```python
from build123d import *

# Parameters (mm, degrees)
F1_DEPTH = 2.5
F2_R     = 0.5
F3_DEPTH = 25


with BuildPart() as f1:
    # F0 (on Front) → F1 (new body, symmetric)
    with BuildSketch(Plane.XZ):
        with BuildLine():
            Line((121.261015, -15), (150, -15))
            ThreePointArc((150, -15), (0, 14.918645), (-150, -15))
            Line((-150, -15), (-121.261015, -15))
            ThreePointArc((-121.261015, -15), (0, 4.565027), (121.261015, -15))
        make_face()
    extrude(amount=F1_DEPTH, both=True)

    # F2 (on Top) → F3 (join)
    with BuildSketch(Plane.XY):
        with Locations((-2, 0)):
            Circle(F2_R)
        with BuildLine():
            ThreePointArc((2.5, 0), (2, 0.5), (1.5, 0))
            ThreePointArc((1.5, 0), (2, -0.5), (2.5, 0))
        make_face()
    extrude(amount=F3_DEPTH)


solid = f1.part
```
Can you work these out from the model? Positions are in its coordinate system, mm. Round coordinates to 2 decimals unless told otherwise and drop trailing zeros. Loops run counter-clockwise (first coordinate to the right, second up) from the corner with the lowest first, then second, coordinate; pieces in that order, holes last.
Item 1: Suppose I cut it at B-B, the plane y = -1.4. Write out the boundary of the cut face in (x, z), then the cut area to 3 significant figures.
Item 2: Suppose I cut it at A-A, the plane z = 19.5. Write out the boundary of the cut face in (x, y), then the cut area to 3 significant figures.
Item 3: If we mould it in two halves opening along X, with no side actions, what happens to faces 1 (the cylindrical face through (-1.727, -0.591, 4.561)), 2 (the flat face through (-1, -2.5, 6))? For each: +X half, -X half, draft (parallel to the pull), parting line (faces both ways), or undercut.
Item 4: Suppose I cut it at C-C, the plane x = -88.5. Write out the boundary of the cut face in (y, z).
Item 5: Please list where these lines run through material, in increasing order: L1, parallel to X at y = 0.3, z = 21; L2, parallel to Z at x = 57, y = 1.9; L3, parallel to Z at x = 44, y = 0.95.
Item 6: Suppose I cut it at D-D, the plane z = -12. Write out the boundary of the cut face in (x, y), then the cut area to 3 significant figures.
Item 7: Will these pins go through, and if not, where does the flat tip stop? pin 1 Ø0.8 at (x, y) = (2, 0) entering from -Z; pin 2 Ø2 at (y, z) = (0.5, 19.5) entering from +X.
Reported:
1. outline: (-150, -15) - (-121.26, -15) arc R385.56 cw to (121.26, -15) - (150, -15) arc R390.98 ccw to start
1. area: 2,850 mm2
2. outline: circle Ø1 at (-2, 0); circle Ø1 at (2, 0)
2. area: 1.57 mm2
3. face 1: undercut
3. face 2: draft
4. outline: (-2.5, -5.73) - (2.5, -5.73) - (2.5, 4.77) - (-2.5, 4.77) - close
5. L1: x = -2.4 to -1.6, 1.6 to 2.4
5. L2: z = 0.33 to 10.74
5. L3: z = 2.05 to 12.43
6. outline: (-142.56, -2.5) - (-111.8, -2.5) - (-111.8, 2.5) - (-142.56, 2.5) - close; (111.8, -2.5) - (142.56, -2.5) - (142.56, 2.5) - (111.8, 2.5) - close
6. area: 308 mm2
7. pin 1: stops at z = 0
7. pin 2: stops at x = 2.5
